```python
from build123d import *

# Parameters (mm, degrees)
SKETCH_1_R          = 1.2
EXTRUDE_1_DEPTH     = 3
EXTRUDE_2_DEPTH     = 133
FILLET_1_R          = 4
SKETCH_4_W          = 29.077288304
SKETCH_4_H          = 31.423180799
CUT_EXTRUDE_1_DEPTH = 4
FILLET_3_R          = 8


with BuildPart() as part:
    # 草图1 → 凸台-拉伸1 (new body)
    with BuildSketch(Plane.XY):
        Polygon((-67.574588252, 2.235418745), (-78.389048292, -19.637108636), (-56.517207821, -30.451229046), (-45.702747781, -8.578701665), align=None)
        with Locations((-66.577549394, -0.711768645)):
            Circle(SKETCH_1_R, mode=Mode.SUBTRACT)
        with Locations((-75.441860902, -18.640069777)):
            Circle(SKETCH_1_R, mode=Mode.SUBTRACT)
        with Locations((-57.51355977, -27.504381286)):
            Circle(SKETCH_1_R, mode=Mode.SUBTRACT)
        with Locations((-48.649248262, -9.576080153)):
            Circle(SKETCH_1_R, mode=Mode.SUBTRACT)
    extrude(amount=EXTRUDE_1_DEPTH)

    # 草图2 → 凸台-拉伸2 (add)
    with BuildSketch(Plane.XY.offset(3)):
        Polygon((-86.606649797, -63.783530386), (-34.098567754, 44.118746329), (-30.501825197, 42.368476928), (-83.00990724, -65.533799787), align=None)
    extrude(amount=EXTRUDE_2_DEPTH)

    # 圆角1
    fillet_1_edges = [part.edges().sort_by_distance(p)[0] for p in [
        (-58.772343801, -15.726452512, 3),
        (-62.358074987, -13.953555126, 3),
    ]]
    fillet(fillet_1_edges, radius=FILLET_1_R)

    # 草图4 → 切除-拉伸1 (cut)
    with BuildSketch(Plane(origin=(-44.928588602, 21.863431321, 0), x_dir=(0, 0, 1), z_dir=(-0.8991856392880848, 0.43756735035658034, 0))):
        with Locations((17.538644152, -79.537886422)):
            Rectangle(SKETCH_4_W, SKETCH_4_H)
    extrude(amount=-CUT_EXTRUDE_1_DEPTH, mode=Mode.SUBTRACT)

    # 圆角3
    fillet_3_edges = [part.edges().sort_by_distance(p)[0] for p in [
        (-71.058520557, -36.403392171, 3),
        (-71.058520557, -36.403392171, 32.077288304),
        (-84.808278518, -64.658665086, 32.077288304),
    ]]
    fillet(fillet_3_edges, radius=FILLET_3_R)


solid = part.part
```
The listing builds one solid part. Answer for the finished solid, in the listing's coordinates (mm). A direction names the side the tool comes from. Round coordinates to 2 decimals unless told otherwise and drop trailing zeros. Order: outer loops, then holes, each group sorted by start corner. A loop starts at its lowest first (then second) coordinate and runs counter-clockwise, first axis right, second up. Notation, with made-up numbers: (14.5, 34.5) - (73.5, 34.5) arc R7 ccw to (73.5, 39.5) - close; hole circle Ø6 at (-16, 86.25). An arc over 180 degrees is marked (long way). Put each result on its own line as item: value. Start each with the question number.
(1) Straight lines are drawn through the part: probe 1 along Z at (x, y) = (-42, 22); probe 2 along Z at (x, y) = (-52.5, -22); probe 3 along Y at (x, z) = (-41, 33.5). For each, find the intervals that lie inside material, in ascending order. Write a range as from..to.
(2) Find section B-B (y = -50.5). Give the vertices of the cut face in (x, z).
(3) Given P1, Ø3, axis at x = -74.5, z = 84, coming from the +Y side; P2, Ø4, axis at x = -57.51, y = -27.5, coming from the +Z side; P3, Ø2.5, axis at x = -67.5, y = -27, coming from the -Z side; P4, Ø1.4, axis at x = -48.65, y = -9.58, coming from the -Z side, each flat-ended and moving along its own axis, determine where each tip first touches the part or whether it passes through.
(4) Find section A-A (z = 47). Give the vertices of the cut face in (x, y), plus the area to 3 significant figures.
(5) For faces 1 (the flat face through (-67, -27, 3)), 2 (the flat face through (-45, 20, 3)), 3 (the flat face through (-53, -19, 3)), determine the directions among +Z, -Z, +X, -X, +Y, -Y from which every point of the face is accessible in a straight line to the end or side of a thin tool.
Reply:
1. probe 1: 3..136
1. probe 2: 0..3
1. probe 3: 20.8..29.94
2. outline: (-80.14, 32.08) - (-75.69, 32.08) - (-75.69, 136) - (-80.14, 136) - close
3. P1: y = -35.82
3. P2: z = 3
3. P3: z = 3
3. P4: through
4. outline: (-86.61, -63.78) - (-83.01, -65.53) - (-30.5, 42.37) - (-34.1, 44.12) - close
4. area: 480 mm^2
5. face 1: -Z, -X, -Y
5. face 2: -Z, +X, +Y
5. face 3: +Z, +X, -Y
